Study the drawing (mm; zero at the part's minimum x, y, z) and answer. Round coordinates to 2 decimals unless told otherwise and drop trailing zeros. Write each loop counter-clockwise with the first axis right and the second up, starting at its lowest first coordinate (ties: lowest second). Pieces come first, ordered by that corner, then holes.
(1) Find the intervals of material crossed by probe 1 along Y at (x, z) = (15, 0.55); probe 2 along X at (y, z) = (14, 0.2); probe 3 along X at (y, z) = (14.25, 0.2), in increasing order.
(2) A cutting plane is placed at D-D, the plane x = 15.5. Give the vertices of the cut face in (y, z).
(3) This flat-tipped pin is pushed along its axis until it touches: pin 1 Ø5 at (x, y) = (15, 15) entering from +Z. Where does it stop, or does it pass through?
(4) A cutting plane is placed at A-A, the plane z = 0.2. Give the vertices of the cut face in (x, y).
(5) A cutting plane is placed at B-B, the plane y = 15. Give the vertices of the cut face in (x, z).
(6) A cutting plane is placed at C-C, the plane x = 34.5. Give the vertices of the cut face in (y, z).
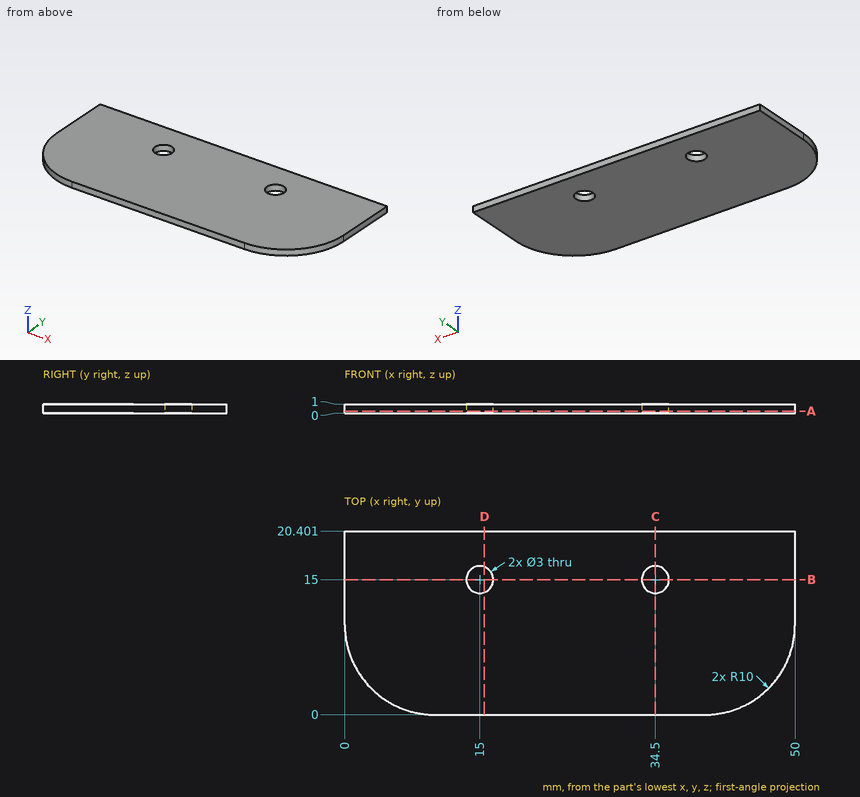
Solutions:
1. probe 1: y = 0 to 13.5, 16.5 to 20.4
1. probe 2: x = 0 to 13.88, 16.12 to 33.38, 35.62 to 50
1. probe 3: x = 0 to 13.7, 16.3 to 33.2, 35.8 to 50
2. outline: (0, 0) - (13.59, 0) - (13.59, 1) - (0, 1) - close; (16.41, 0) - (20.4, 0) - (20.4, 1) - (16.41, 1) - close
3. pin 1: stops at z = 1
4. outline: (0, 10) arc R10 ccw to (10, 0) - (40, 0) arc R10 ccw to (50, 10) - (50, 20.4) - (0, 20.4) - close; hole circle Ø3 at (15, 15); hole circle Ø3 at (34.5, 15)
5. outline: (0, 0) - (13.5, 0) - (13.5, 1) - (0, 1) - close; (16.5, 0) - (33, 0) - (33, 1) - (16.5, 1) - close; (36, 0) - (50, 0) - (50, 1) - (36, 1) - close
6. outline: (0, 0) - (13.5, 0) - (13.5, 1) - (0, 1) - close; (16.5, 0) - (20.4, 0) - (20.4, 1) - (16.5, 1) - close
